For this review, take the finished solid that the model builds, in its own axes (mm). A direction names the side the tool comes from. Coordinates: 2 decimals unless noted, no trailing zeros. Loops run counter-clockwise (first coordinate to the right, second up) from the corner with the lowest first, then second, coordinate; pieces in that order, holes last. Notation, with made-up numbers: (89, 76.5) -> (107, 76.5) arc R14 cw to (107, 92.5) -> close; hole circle Ø8 at (0.25, -1). An arc over 180 degrees is marked (long way). Use a Markdown table: item, result.
from build123d import *

# Parameters (mm, degrees)
PAD_DEPTH    = 75
CHAMFER_SIZE = 1


with BuildPart() as part:
    # Sketch → Pad (new body)
    with BuildSketch(Plane.XY):
        with BuildLine():
            Line((4, 27), (4, 10))
            Line((4, 10), (16, 10))
            ThreePointArc((17.55441, 6.741505), (17.80513, 8.861107), (16, 10))
            Line((17.55441, 6.741505), (4, -10))
            Line((4, -10), (4, -29.001949))
            ThreePointArc((4, -29.001949), (5.550868, -30.950867), (7.798281, -29.87727))
            Line((7.798281, -29.87727), (26.843334, 9.249358))
            ThreePointArc((26.843334, 9.249358), (26.638127, 13.121018), (23.246773, 15))
            Line((15, 15), (23.246773, 15))
            ThreePointArc((11, 19), (12.171573, 16.171573), (15, 15))
            Line((11, 27), (11, 19))
            ThreePointArc((11, 27), (7.5, 30.5), (4, 27))
        make_face()
    extrude(amount=PAD_DEPTH)

    # Chamfer
    chamfer_edges = [part.edges().sort_by_distance(p)[0] for p in [
        (7.5, 30.5, 75),
        (4, 18.5, 75),
        (10, 10, 75),
        (17.80513, 8.861107, 75),
        (10.777205, -1.629248, 75),
        (4, -19.500975, 75),
        (5.550868, -30.950867, 75),
        (17.320807, -10.313956, 75),
        (26.638127, 13.121018, 75),
        (19.123386, 15, 75),
        (12.171573, 16.171573, 75),
        (11, 23, 75),
        (7.5, 30.5, 0),
        (4, 18.5, 0),
        (10, 10, 0),
        (17.80513, 8.861107, 0),
        (10.777205, -1.629248, 0),
        (4, -19.500975, 0),
        (5.550868, -30.950867, 0),
        (17.320807, -10.313956, 0),
        (26.638127, 13.121018, 0),
        (19.123386, 15, 0),
        (12.171573, 16.171573, 0),
        (11, 23, 0),
    ]]
    chamfer(chamfer_edges, length=CHAMFER_SIZE)


solid = part.part
(1) Take a section at A-A on z = 23. Write out the cut boundary in (x, y).
Found:
| item | result |
|---|---|
| outline | (4, -29) arc R2 ccw to (7.8, -29.88) -> (26.84, 9.25) arc R4 ccw to (23.25, 15) -> (15, 15) arc R4 cw to (11, 19) -> (11, 27) arc R3.5 ccw to (4, 27) -> (4, 10) -> (16, 10) arc R2 cw to (17.55, 6.74) -> (4, -10) -> close |
(2) Mouldability with a two-part tool opening along Y and no side actions: class faces 1 (the face through (18.046, 9.016, 74.285)), 2 (the face through (6, -31, 37)), 3 (the face through (7.6, 29.7, 74.8)) as pulls with the +Y half, pulls with the -Y half, needs draft (parallel to the pull), parting line crosses it, or undercut.
Found:
| item | result |
|---|---|
| face 1 | undercut |
| face 2 | pulls with the -Y half |
| face 3 | pulls with the +Y half |
(3) For faces 4 (the face through (11, 23, 37)), 5 (the face through (10.872, -1.512, 36.989)), 6 (the face through (11.27, -1.83, 0.49)), 7 (the face through (15, 0, 0)), list the 3-axis set-ups (+Z, -Z, +X, -X, +Y, -Y) from which the entire face can be reached by the end or side of a thin tool; tool diameter is ignored.
Found:
| item | result |
|---|---|
| face 4 | +Z, -Z, +X, +Y |
| face 5 | +Z, -Z, -X |
| face 6 | -Z, -X |
| face 7 | -Z, +X, -X, +Y, -Y |
(4) Take a section at C-C on y = 4. Write out the cut boundary in (x, z), plus the area to 3 significant figures.
Found:
| item | result |
|---|---|
| outline | (15.33, 1) -> (16.62, 0) -> (23.18, 0) -> (24.29, 1) -> (24.29, 74) -> (23.18, 75) -> (16.62, 75) -> (15.33, 74) -> close |
| area | 669 mm^2 |
(5) Take a section at B-B on y = -3. Write out the cut boundary in (x, z).
Found:
| item | result |
|---|---|
| outline | (9.67, 1) -> (10.95, 0) -> (19.77, 0) -> (20.88, 1) -> (20.88, 74) -> (19.77, 75) -> (10.95, 75) -> (9.67, 74) -> close |
(6) For line 1 along X through (y, z) = (23, 13); line 2 along Y through (x, z) = (7.25, 3); line 3 along Y through (x, z) = (8.25, 19), list the stretches that pass through material, from the lowest coordinate up.
Found:
| item | result |
|---|---|
| line 1 | x = 4 to 11 |
| line 2 | y = -30.56 to -5.99, 10 to 30.49 |
| line 3 | y = -28.95 to -4.75, 10 to 30.42 |
(7) For pin 1 Ø1.5 at (x, z) = (17.5, 45) entering from -Y; pin 2 Ø6.5 at (x, z) = (18.5, 35) entering from +Y; pin 3 Ø6 at (x, z) = (9, 56) entering from -Y; pin 4 Ø1.5 at (x, z) = (16, 63) entering from -Y, all flat-tipped, find the tip position at first contact; note any pin that passes through.
Found:
| item | result |
|---|---|
| pin 1 | stops at y = -11.49 |
| pin 2 | stops at y = 15 |
| pin 3 | stops at y = -31 |
| pin 4 | stops at y = -14.57 |
